from build123d import *

# Parameters (mm, degrees)
SKETCH1_W           = 170
SKETCH1_H           = 80
BOSS_EXTRUDE1_DEPTH = 7
SKETCH2_W           = 7
SKETCH2_H           = 18
BOSS_EXTRUDE2_DEPTH = 18
SKETCH3_R           = 2
CUT_EXTRUDE1_DEPTH  = 20
SKETCH4_W           = 7
SKETCH4_H           = 8
CUT_EXTRUDE2_DEPTH  = 2.3
SKETCH5_W           = 150
SKETCH5_H           = 22.295371368
CUT_EXTRUDE3_DEPTH  = 11
SKETCH6_R           = 2
SKETCH6_W           = 20
SKETCH6_H           = 20.5
CUT_EXTRUDE4_DEPTH  = 11
SKETCH7_R           = 2
CUT_EXTRUDE5_DEPTH  = 25
SKETCH7_2_R         = 2
CUT_EXTRUDE6_DEPTH  = 25
SKETCH10_R          = 2
CUT_EXTRUDE7_DEPTH  = 10


with BuildPart() as part:
    # Sketch1 → Boss-Extrude1 (new body)
    with BuildSketch(Plane(origin=(0, 0, 0), x_dir=(1, 0, 0), z_dir=(0, 1, 0))):
        with Locations((5.170316302, -0.291970803)):
            Rectangle(SKETCH1_W, SKETCH1_H)
    extrude(amount=BOSS_EXTRUDE1_DEPTH)

    # Sketch2 → Boss-Extrude2 (add)
    with BuildSketch(Plane(origin=(0, 7, 0), x_dir=(1, 0, 0), z_dir=(0, 1, 0))):
        with Locations((-76.329683698, -0.291970803)):
            Rectangle(SKETCH2_W, SKETCH2_H)
    extrude(amount=BOSS_EXTRUDE2_DEPTH)

    # Sketch3 → Cut-Extrude1 (cut)
    with BuildSketch(Plane(origin=(0, 0, -8.708029197), x_dir=(-1, 0, 0), z_dir=(0, 0, -1))):
        with Locations((76.329683698, 17)):
            Circle(SKETCH3_R)
    extrude(amount=-CUT_EXTRUDE1_DEPTH, mode=Mode.SUBTRACT)

    # Sketch4 → Cut-Extrude2 (cut)
    with BuildSketch(Plane.XY.offset(9.291970803)):
        with Locations((-76.329683698, 17)):
            Rectangle(SKETCH4_W, SKETCH4_H)
    extrude(amount=-CUT_EXTRUDE2_DEPTH, mode=Mode.SUBTRACT)

    # Sketch5 → Cut-Extrude3 (cut)
    with BuildSketch(Plane(origin=(0, 7, 0), x_dir=(1, 0, 0), z_dir=(0, 1, 0))):
        with Locations((5.170316302, -24.144285119)):
            Rectangle(SKETCH5_W, SKETCH5_H)
    extrude(amount=-CUT_EXTRUDE3_DEPTH, mode=Mode.SUBTRACT)

    # Sketch6 → Cut-Extrude4 (cut)
    with BuildSketch(Plane(origin=(0, 7, 0), x_dir=(1, 0, 0), z_dir=(0, 1, 0))):
        with Locations((86.170316302, -26.191970803)):
            Circle(SKETCH6_R)
        with Locations((80.170316302, 9.958029197)):
            Rectangle(SKETCH6_W, SKETCH6_H)
    extrude(amount=-CUT_EXTRUDE4_DEPTH, mode=Mode.SUBTRACT)

    # Sketch7 → Cut-Extrude5 (cut)
    with BuildSketch(Plane.XY.offset(-20.208029197)):
        with Locations((80.170316302, 3.5)):
            Circle(SKETCH7_R)
    extrude(amount=-CUT_EXTRUDE5_DEPTH, mode=Mode.SUBTRACT)

    # Sketch7_2 → Cut-Extrude6 (cut)
    with BuildSketch(Plane.XY.offset(-20.208029197)):
        with Locations((80.170316302, 3.5)):
            Circle(SKETCH7_2_R)
    extrude(amount=CUT_EXTRUDE6_DEPTH, mode=Mode.SUBTRACT)

    # Sketch10 → Cut-Extrude7 (cut)
    with BuildSketch(Plane.XZ):
        with Locations((-39.829683698, -9.708029197)):
            Circle(SKETCH10_R)
        with Locations((-39.829683698, -24.708029197)):
            Circle(SKETCH10_R)
        with Locations((-14.829683698, -24.708029197)):
            Circle(SKETCH10_R)
        with Locations((-14.829683698, -9.708029197)):
            Circle(SKETCH10_R)
    extrude(amount=-CUT_EXTRUDE7_DEPTH, mode=Mode.SUBTRACT)


solid = part.part
Verification items for the finished model (mm, model axes). A direction names the side the tool comes from. Round coordinates to 2 decimals unless told otherwise and drop trailing zeros. Order: outer loops, then holes, each group sorted by start corner. A loop starts at its lowest first (then second) coordinate and runs counter-clockwise, first axis right, second up. Notation, with made-up numbers: (48, -26.5) -> (96, -26.5) arc R32 ccw to (96, 11.5) -> close; hole circle Ø8 at (65.5, -24.5). An arc over 180 degrees is marked (long way). Put each result on its own line as item: value.
1) Mould release check, pull along Y, two halves, no side actions. Record for faces 4 (the flat face through (-76, 25, 0)), 5 (the cylindrical face through (82.08, 4.1, -29.82)), 6 (the flat face through (-69.83, 4, 24)): +Y half, -Y half, draft (parallel to the pull), parting line (faces both ways), or undercut.
Final values:
face 4: +Y half
face 5: undercut
face 6: draft
2) Depth check by flat-ended pin: pin 1 (3 mm diameter, centred on x = 80.17, y = 3.5, fed in from -Z); pin 2 (9 mm diameter, centred on y = 18, z = -2.5, fed in from +X); pin 3 (7.5 mm diameter, centred on x = -75, y = 17.5, fed in from -Z). Enter the tip coordinate at first touch or a pass-through.
Final values:
pin 1: stops at z = 4.79
pin 2: stops at x = -72.83
pin 3: stops at z = -8.71
3) Section check C-C (y = 3.5). Record the cut outline in (x, z), then the cut area to 3 significant figures.
Final values:
outline: (-79.83, -39.71) -> (78.17, -39.71) -> (78.17, -20.21) -> (70.17, -20.21) -> (70.17, 0.29) -> (78.17, 0.29) -> (78.17, 4.79) -> (82.17, 4.79) -> (82.17, 0.29) -> (90.17, 0.29) -> (90.17, 40.29) -> (-79.83, 40.29) -> close; (82.17, -39.71) -> (90.17, -39.71) -> (90.17, -20.21) -> (82.17, -20.21) -> close; hole (-69.83, 13) -> (80.17, 13) -> (80.17, 35.29) -> (-69.83, 35.29) -> close; hole circle Ø4 at (-39.83, -24.71); hole circle Ø4 at (-39.83, -9.71); hole circle Ø4 at (-14.83, -24.71); hole circle Ø4 at (-14.83, -9.71); hole circle Ø4 at (86.17, 26.19)
area: 9,690 mm^2
4) Section check B-B (x = 38). Record the cut outline in (y, z), then the cut area to 3 significant figures.
Final values:
outline: (0, -39.71) -> (7, -39.71) -> (7, 13) -> (0, 13) -> close; (0, 35.29) -> (7, 35.29) -> (7, 40.29) -> (0, 40.29) -> close
area: 404 mm^2
5) Material ranges on line 1 (Z direction, x = -37, y = 5.75); line 2 (X direction, y = 2.5, z = -7); line 3 (Y direction, x = 65, z = 4.5), recorded low to high.
Final values:
line 1: z = -39.71 to 13, 35.29 to 40.29
line 2: x = -79.83 to 70.17
line 3: y = 0 to 7
6) Section check A-A (z = 32). Record the cut outline in (x, y), then the cut area to 3 significant figures.
Final values:
outline: (-79.83, 0) -> (-69.83, 0) -> (-69.83, 7) -> (-79.83, 7) -> close; (80.17, 0) -> (90.17, 0) -> (90.17, 7) -> (80.17, 7) -> close
area: 140 mm^2
7) Set-up check for faces 1 (the flat face through (80, 4, 4.792)), 2 (the flat face through (4, 4, 35.292)), 3 (the flat face through (-76, 23, 9.292)): record each of +Z, -Z, +X, -X, +Y, -Y from which the full face is reachable in a straight line by a thin tool's end or side.
Final values:
face 1: -Z
face 2: +Y, -Y
face 3: +Z, +X, -X, +Y
